Check sheet for the modelled part. Datum: model origin and axes. Units: mm. Face numbers are marked on the shaded views. A direction names the side the tool comes from. Give positions to 0.01 mm unless a question says otherwise; leave off trailing zeros. Write each loop counter-clockwise with the first axis right and the second up, starting at its lowest first coordinate (ties: lowest second). Pieces come first, ordered by that corner, then holes. Notation, with made-up numbers: (11, 79.5) -> (55, 79.5) arc R17 ccw to (55, 96.5) -> close; hole circle Ø11 at (60, 82.5). An arc over 180 degrees is marked (long way). Use a Markdown table: item, result. Add a question column.
1. Gauge pin test, flat ends, axial feed: P1, Ø3, axis at x = -25, y = 4, coming from the +Z side; P2, Ø9.5, axis at x = -25, y = 3, coming from the +Z side. Record the tip position at first contact, or that the pin passes through.
2. Scan lines: probe 1 along Y at (x, z) = (25, 6.5); probe 2 along Y at (x, z) = (0, 9.5); probe 3 along X at (y, z) = (-1, 5.5). Record each from-to range of solid material in increasing order. Write a range as [from, to].
3. Set-up check for the marked faces 4 and 5: record each of +Z, -Z, +X, -X, +Y, -Y from which the full face is reachable in a straight line by a thin tool's end or side.
4. Cross-section at A-A (x = -25). Enter the section's corners in (y, z).
5. Cross-section at B-B (y = 3). Enter the section's corners in (x, z).
6. Cross-section at D-D (x = 0). Enter the section's corners in (y, z), then the cut area to 3 significant figures.
7. Cross-section at C-C (z = 8.5). Enter the section's corners in (x, y), then the cut area to 3 significant figures.
8. Release check for a two-part mould opening along Y. For the marked faces 1, 2 and 3 record: released by +Y, released by -Y, zero draft, split by the parting line, or undercut.
from build123d import *

# Parameters (mm, degrees)
SKETCH_W     = 85
SKETCH_H     = 18
SKETCH_R     = 5
SKETCH_R_2   = 3.2
PAD_DEPTH    = 16
SKETCH001_R  = 5.4
POCKET_DEPTH = 5


with BuildPart() as part:
    # Sketch → Pad (new body)
    with BuildSketch(Plane.XY):
        Rectangle(SKETCH_W, SKETCH_H)
        Circle(SKETCH_R, mode=Mode.SUBTRACT)
        with Locations((-25, 3)):
            Circle(SKETCH_R_2, mode=Mode.SUBTRACT)
        with Locations((25, 3)):
            Circle(SKETCH_R_2, mode=Mode.SUBTRACT)
    extrude(amount=PAD_DEPTH)

    # Sketch001 → Pocket (cut)
    with BuildSketch(Plane.XY.offset(16)):
        with Locations((-25, 3)):
            Circle(SKETCH001_R)
        with Locations((25, 3)):
            Circle(SKETCH001_R)
    extrude(amount=-POCKET_DEPTH, mode=Mode.SUBTRACT)


solid = part.part
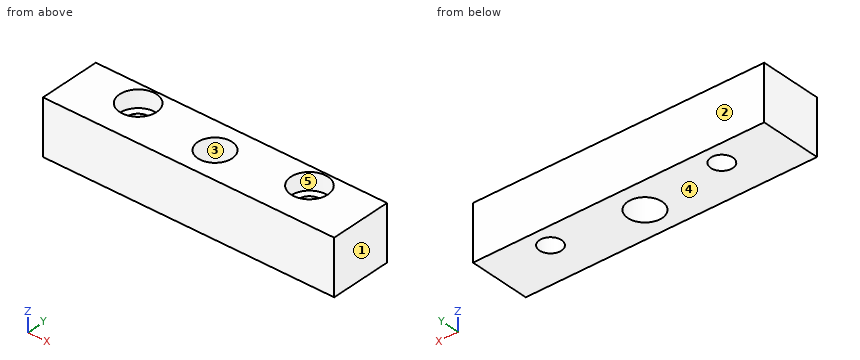
Worked answers:
| question | item | result |
|---|---|---|
| 1 | P1 | passes through |
| 1 | P2 | stops at z = 11 |
| 2 | probe 1 | y = [-9, -0.2], [6.2, 9] |
| 2 | probe 2 | y = [-9, -5], [5, 9] |
| 2 | probe 3 | x = [-42.5, -4.9], [4.9, 42.5] |
| 3 | face 4 | -Z, +X, -X, +Y, -Y |
| 3 | face 5 | +Z |
| 4 | outline | (-9, 0) -> (-0.2, 0) -> (-0.2, 11) -> (-2.4, 11) -> (-2.4, 16) -> (-9, 16) -> close; (6.2, 0) -> (9, 0) -> (9, 16) -> (8.4, 16) -> (8.4, 11) -> (6.2, 11) -> close |
| 5 | outline | (-42.5, 0) -> (-28.2, 0) -> (-28.2, 11) -> (-30.4, 11) -> (-30.4, 16) -> (-42.5, 16) -> close; (-21.8, 0) -> (-4, 0) -> (-4, 16) -> (-19.6, 16) -> (-19.6, 11) -> (-21.8, 11) -> close; (4, 0) -> (21.8, 0) -> (21.8, 11) -> (19.6, 11) -> (19.6, 16) -> (4, 16) -> close; (28.2, 0) -> (42.5, 0) -> (42.5, 16) -> (30.4, 16) -> (30.4, 11) -> (28.2, 11) -> close |
| 6 | outline | (-9, 0) -> (-5, 0) -> (-5, 16) -> (-9, 16) -> close; (5, 0) -> (9, 0) -> (9, 16) -> (5, 16) -> close |
| 6 | area | 128 mm² |
| 7 | outline | (-42.5, -9) -> (42.5, -9) -> (42.5, 9) -> (-42.5, 9) -> close; hole circle Ø6.4 at (-25, 3); hole circle Ø10 at (0, 0); hole circle Ø6.4 at (25, 3) |
| 7 | area | 1,390 mm² |
| 8 | face 1 | zero draft |
| 8 | face 2 | released by +Y |
| 8 | face 3 | undercut |
